Check sheet for the modelled part. Datum: model origin and axes. Units: mm. A direction names the side the tool comes from. Give positions to 0.01 mm unless a question says otherwise; leave off trailing zeros. Write each loop counter-clockwise with the first axis right and the second up, starting at its lowest first coordinate (ties: lowest second). Pieces come first, ordered by that corner, then holes. Notation, with made-up numbers: M -39,-24.75 L -25,-24.75 A21 cw -25,13.25 Z; hole C 47.5,79 d8. An arc over 180 degrees is marked long. One line per item, written item: value. Start each with the question number.
from build123d import *

# Parameters (mm, degrees)
SKETCH1_R           = 5
BOSS_EXTRUDE1_DEPTH = 250
CUT_EXTRUDE1_START  = 5
SKETCH5_R           = 2.5
CUT_EXTRUDE1_DEPTH  = 2


with BuildPart() as part:
    # Sketch1 → Boss-Extrude1 (new body)
    with BuildSketch(Plane(origin=(0, 0, 0), x_dir=(1, 0, 0), z_dir=(0, 1, 0))):
        with Locations(Location((0, 0, 0), (0, 0, 270))):
            Circle(SKETCH1_R)
    extrude(amount=BOSS_EXTRUDE1_DEPTH)

    # Sketch5 → Cut-Extrude1 (cut)
    with BuildSketch(Plane.XY.offset(CUT_EXTRUDE1_START)):
        with Locations((0, 5)):
            Circle(SKETCH5_R)
        with Locations((0, 20)):
            Circle(SKETCH5_R)
        with Locations((0, 245)):
            Circle(SKETCH5_R)
        with Locations((0, 230)):
            Circle(SKETCH5_R)
    extrude(amount=-CUT_EXTRUDE1_DEPTH, mode=Mode.SUBTRACT)


solid = part.part
1) Draft check along Y on faces 1 (the flat face through (0, 0, 0)), 2 (the cylindrical face through (-2.5, 230.1, 3.8)), 3 (the flat face through (0, 250, 0)). Enter one of: released by +Y, released by -Y, zero draft, split by the parting line, or undercut.
2) Material ranges on L1, parallel to Y at x = 0, z = 3.55; L2, parallel to X at y = 230, z = 3.5; L3, parallel to X at y = 5, z = 3.6, recorded low to high. Write a range as from..to.
3) Tool access check on faces 4 (the flat face through (0, 245, 3)), 5 (the cylindrical face through (-4.88, 123.25, -1.08)). Record the directions out of +Z, -Z, +X, -X, +Y, -Y that give a thin tool (end or side, any length) a straight path to the whole face; none if there is none.
4) Cross-section at C-C (y = 245). Record the boundary of the cut face in (x, z), plus the area to 3 significant figures.
5) Cross-section at B-B (y = 132.5). Record the boundary of the cut face in (x, z), plus the area to 3 significant figures.
6) Cross-section at A-A (x = 0). Record the boundary of the cut face in (y, z), plus the area to 3 significant figures.
7) Gauge pin test, flat ends, axial feed: pin 1 (1.5 mm diameter, centred on x = 0, y = 244.5, fed in from +Z); pin 2 (3 mm diameter, centred on x = 2.5, y = 165, fed in from +Z). Record the tip position at first contact, or that the pin passes through.
Data:
1. face 1: released by -Y
1. face 2: undercut
1. face 3: released by +Y
2. L1: y = 0..2.5, 7.5..17.5, 22.5..227.5, 232.5..242.5, 247.5..250
2. L2: x = -3.57..-2.5, 2.5..3.57
2. L3: x = -3.47..-2.5, 2.5..3.47
3. face 4: +Z
3. face 5: +Y, -Y
4. outline: M -2.5,3 L -2.5,4.33 A5 ccw long 2.5,4.33 L 2.5,3 Z
4. area: 69.6 mm2
5. outline: C 0,0 d10
5. area: 78.5 mm2
6. outline: M 0,-5 L 250,-5 L 250,5 L 247.5,5 L 247.5,3 L 242.5,3 L 242.5,5 L 232.5,5 L 232.5,3 L 227.5,3 L 227.5,5 L 22.5,5 L 22.5,3 L 17.5,3 L 17.5,5 L 7.5,5 L 7.5,3 L 2.5,3 L 2.5,5 L 0,5 Z
6. area: 2,460 mm2
7. pin 1: stops at z = 3
7. pin 2: stops at z = 4.9
